```python
from build123d import *

# Parameters (mm, degrees)
EXTRUDE_1_DEPTH = 290
FILLET_1_R      = 1


with BuildPart() as part:
    # Эскиз1 → Бобышка-Вытянуть1 (new body)
    with BuildSketch(Plane.XY):
        Polygon((0, 0), (0, 20), (20, 0), align=None)
    extrude(amount=-EXTRUDE_1_DEPTH)

    # Скругление1
    fillet_1_edges = [part.edges().sort_by_distance(p)[0] for p in [
        (0, 20, -145),
        (20, 0, -145),
    ]]
    fillet(fillet_1_edges, radius=FILLET_1_R)


solid = part.part
```
Geometry check sheet. Reference: the model listing, model coordinates, mm. Coordinates: 2 decimals unless noted, no trailing zeros. Order: outer loops, then holes, each group sorted by start corner. A loop starts at its lowest first (then second) coordinate and runs counter-clockwise, first axis right, second up.
Item 1: Scan lines: line 1 along X through (y, z) = (1.25, -250); line 2 along X through (y, z) = (11, -202); line 3 along Y through (x, z) = (10.5, -27.5). Record each from-to range of solid material in increasing order.
Item 2: Section check C-C (x = 11.5). Enter the section's corners in (y, z), plus the area to 4 significant figures.
Item 3: Depth check by flat-ended pin: pin 1 (1.5 mm diameter, centred on x = 3, z = -138.5, fed in from +Y); pin 2 (3 mm diameter, centred on y = 2.5, z = -206.5, fed in from +X); pin 3 (4 mm diameter, centred on y = 6, z = -153, fed in from +X); pin 4 (2 mm diameter, centred on y = 13.5, z = -247.5, fed in from +X). Enter the tip coordinate at first touch or a pass-through.
Item 4: Section check A-A (z = -198.5). Enter the section's corners in (x, y), plus the area to 3 significant figures.
Item 5: Section check B-B (y = 15). Enter the section's corners in (x, z), plus the area to 3 significant figures.
Check sheet entries:
1. line 1: x = 0 to 18.55
1. line 2: x = 0 to 9
1. line 3: y = 0 to 9.5
2. outline: (0, -290) - (8.5, -290) - (8.5, 0) - (0, 0) - close
2. area: 2,465 mm2
3. pin 1: stops at y = 17.75
3. pin 2: stops at x = 18.59
3. pin 3: stops at x = 16
3. pin 4: stops at x = 7.5
4. outline: (0, 0) - (17.59, 0) arc R1 ccw to (18.29, 1.71) - (1.71, 18.29) arc R1 ccw to (0, 17.59) - close
4. area: 198 mm2
5. outline: (0, -290) - (5, -290) - (5, 0) - (0, 0) - close
5. area: 1,450 mm2
